```python
from build123d import *

# Parameters (mm, degrees)
SKETCH1_W           = 99
SKETCH1_H           = 199
BOSS_EXTRUDE1_DEPTH = 30
SKETCH2_W           = 99
SKETCH2_H           = 198.99569364
BOSS_EXTRUDE2_DEPTH = 200
FILLET1_R           = 100
SKETCH3_R           = 85
CUT_EXTRUDE1_DEPTH  = 99


with BuildPart() as part:
    # Sketch1 → Boss-Extrude1 (new body)
    with BuildSketch(Plane(origin=(0, 0, 0), x_dir=(1, 0, 0), z_dir=(0, 1, 0))):
        Rectangle(SKETCH1_W, SKETCH1_H)
    extrude(amount=BOSS_EXTRUDE1_DEPTH)

    # Sketch2 → Boss-Extrude2 (add)
    with BuildSketch(Plane(origin=(0, 30, 0), x_dir=(1, 0, 0), z_dir=(0, 1, 0))):
        Rectangle(SKETCH2_W, SKETCH2_H)
    extrude(amount=BOSS_EXTRUDE2_DEPTH)

    # Fillet1
    # the kernel refuses this fillet: 100 mm, written as the material it takes off along each edge
    with BuildSketch(Plane(origin=(-299.5, 230, -99.49784682), x_dir=(0, -1, 0), z_dir=(1, 0, 0)), Plane(origin=(299.5, 230, 99.49784682), x_dir=(0, -1, 0), z_dir=(-1, 0, 0))) as fillet1_piece_1:
        with BuildLine():
            CenterArc((FILLET1_R, -FILLET1_R), FILLET1_R, 90, 90)
            Line((0, -FILLET1_R), (0, 0))
            Line((0, 0), (FILLET1_R, 0))
        make_face()
    extrude(amount=599, mode=Mode.SUBTRACT)

    # Sketch3 → Cut-Extrude1 (cut)
    with BuildSketch(Plane(origin=(49.5, 0, 0), x_dir=(0, 0, -1), z_dir=(1, 0, 0))):
        with Locations((0.50215318, 130)):
            Circle(SKETCH3_R)
    extrude(amount=-CUT_EXTRUDE1_DEPTH, mode=Mode.SUBTRACT)


solid = part.part
```
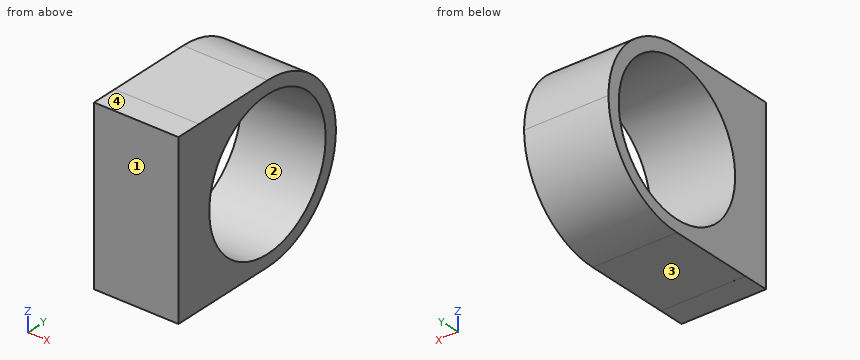
Build history of the part. All positions in model axes, mm. Face numbers are marked on the shaded views. Coordinates: 2 decimals unless noted, no trailing zeros. Write each loop counter-clockwise with the first axis right and the second up, starting at its lowest first coordinate (ties: lowest second). Pieces come first, ordered by that corner, then holes.
1. Band-saw the part on B-B, the plane z = 78.5. Give the cut face in (x, y).
Answer block:
outline: (-49.5, 0) - (49.5, 0) - (49.5, 98.64) - (-49.5, 98.64) - close; (-49.5, 161.36) - (49.5, 161.36) - (49.5, 191.31) - (-49.5, 191.31) - close
2. Drill centre lines: probe 1 along Y at (x, z) = (-41.5, 24); probe 2 along Y at (x, z) = (-2, 71); probe 3 along Z at (x, y) = (41, 133.5). Where is each one in solid material? Low to high.
Answer block:
probe 1: y = 0 to 48.61, 211.39 to 226.95
probe 2: y = 0 to 84.04, 175.96 to 199.91
probe 3: z = -99.44 to -85.43, 84.43 to 99.44
3. Drop flat-ended pins along their axis: pin 1 (6 mm diameter, centred on x = 16.5, y = 46, fed in from -Z); pin 2 (2 mm diameter, centred on x = -33.5, y = 201.5, fed in from -Z); pin 3 (4 mm diameter, centred on x = -11, y = 45.5, fed in from +Z). Give the stop position or say it passes through.
Answer block:
pin 1: stops at z = -99.5
pin 2: stops at z = -70.42
pin 3: stops at z = 99.5
4. Pull direction Z, two halves, no side cores. Call the marked faces 1, 2, 3 and 4: released by +Z, released by -Z, zero draft, split by the parting line, or undercut.
Answer block:
face 1: zero draft
face 2: undercut
face 3: released by -Z
face 4: released by +Z
5. Band-saw the part on A-A, the plane y = 110. Give the cut face in (x, z), and give its area (3 significant figures).
Answer block:
outline: (-49.5, -99.5) - (49.5, -99.5) - (49.5, -83.12) - (-49.5, -83.12) - close; (-49.5, 82.11) - (49.5, 82.11) - (49.5, 99.5) - (-49.5, 99.5) - close
area: 3,340 mm2
